Can you work these out from the model? Positions are in its coordinate system, mm. A direction names the side the tool comes from. Give positions to 0.01 mm unless a question says otherwise; leave off trailing zeros. Order: outer loops, then holes, each group sorted by start corner. A loop starts at its lowest first (then second) coordinate and runs counter-clockwise, first axis right, second up. Notation, with made-up numbers: (56.25, 50.25) -> (105.25, 50.25) arc R26 cw to (105.25, 83.25) -> close; hole circle Ø7 at (57.5, 79.5). An arc over 180 degrees is marked (long way). Answer as a JSON object with one key per item and string values.
```python
from build123d import *

# Parameters (mm, degrees)
SKETCH1_W                       = 24.8412
SKETCH1_H                       = 46.101
SKETCH1_R                       = 2.6416
BOSS_EXTRUDE1_DEPTH             = 2.54
BOSS_EXTRUDE2_REACH             = 28.307
SKETCH2_R                       = 3.175
BOSS_EXTRUDE2_DIRECTION_2_REACH = 28.307
CUT_EXTRUDE1_DEPTH              = 46.500059073
CUT_EXTRUDE1_DEPTH_BACK         = 46.500059073
SKETCH3_W                       = 19.7612
SKETCH3_H                       = 34.671
FILLET1_R                       = 2.54


with BuildPart() as part:
    # Sketch1 → Boss-Extrude1 (new body)
    with BuildSketch(Plane(origin=(0, 0, 0), x_dir=(1, 0, 0), z_dir=(0, 1, 0))):
        Rectangle(SKETCH1_W, SKETCH1_H)
        with Locations(Location((-8.255, 17.9959, 0), (0, 0, 270))):
            Circle(SKETCH1_R, mode=Mode.SUBTRACT)
        with Locations(Location((8.255, 17.9959, 0), (0, 0, 270))):
            Circle(SKETCH1_R, mode=Mode.SUBTRACT)
        with Locations(Location((8.255, -17.9959, 0), (0, 0, 270))):
            Circle(SKETCH1_R, mode=Mode.SUBTRACT)
        with Locations(Location((-8.255, -17.9959, 0), (0, 0, 270))):
            Circle(SKETCH1_R, mode=Mode.SUBTRACT)
    extrude(amount=-BOSS_EXTRUDE1_DEPTH)

    # Boss-Extrude2: up to this face of the body (flat: up to its plane)
    boss_extrude2_end = Plane(part.part.faces().sort_by_distance((12.4206, -1.27, 0))[0])
    # Sketch2 → Boss-Extrude2 (add, up to the picked face)
    with BuildSketch(Plane(origin=(0, 0, 0), x_dir=(0, 0, -1), z_dir=(1, 0, 0)), mode=Mode.PRIVATE) as boss_extrude2_sk1:
        with BuildLine():
            Line((-6.203113115, -32.218898258), (-12.7, -2.54))
            Line((-12.7, -2.54), (12.7, -2.54))
            Line((12.7, -2.54), (6.203113115, -32.218898258))
            ThreePointArc((6.203113115, -32.218898258), (0, -37.211), (-6.203113115, -32.218898258))
        make_face()
        with Locations(Location((0, -30.861, 0), (0, 0, 180))):
            Circle(SKETCH2_R, mode=Mode.SUBTRACT)
    boss_extrude2_tool1 = split(extrude(boss_extrude2_sk1.sketch, amount=BOSS_EXTRUDE2_REACH, mode=Mode.PRIVATE), bisect_by=boss_extrude2_end, keep=Keep.BOTH, mode=Mode.PRIVATE)
    add(boss_extrude2_tool1.solids().sort_by(Axis((0, -16.339772, 0), (1, 0, 0)))[0])

    # Boss-Extrude2 direction 2: up to this face of the body (flat: up to its plane)
    boss_extrude2_direction_2_end = Plane(part.part.faces().sort_by_distance((-12.4206, -1.27, 0))[0])
    # Sketch2 → Boss-Extrude2 direction 2 (add, up to the picked face)
    with BuildSketch(Plane(origin=(0, 0, 0), x_dir=(0, 0, -1), z_dir=(1, 0, 0)), mode=Mode.PRIVATE) as boss_extrude2_direction_2_sk1:
        with BuildLine():
            Line((-6.203113115, -32.218898258), (-12.7, -2.54))
            Line((-12.7, -2.54), (12.7, -2.54))
            Line((12.7, -2.54), (6.203113115, -32.218898258))
            ThreePointArc((6.203113115, -32.218898258), (0, -37.211), (-6.203113115, -32.218898258))
        make_face()
        with Locations(Location((0, -30.861, 0), (0, 0, 180))):
            Circle(SKETCH2_R, mode=Mode.SUBTRACT)
    boss_extrude2_direction_2_tool1 = split(extrude(boss_extrude2_direction_2_sk1.sketch, amount=-BOSS_EXTRUDE2_DIRECTION_2_REACH, mode=Mode.PRIVATE), bisect_by=boss_extrude2_direction_2_end, keep=Keep.BOTH, mode=Mode.PRIVATE)
    add(boss_extrude2_direction_2_tool1.solids().sort_by(Axis((0, -16.339772, 0), (-1, 0, 0)))[0])

    # Sketch3 → Cut-Extrude1 (cut, two sides: drawn at the far end of the back side and taken through both)
    with BuildSketch(Plane.XY.offset(-CUT_EXTRUDE1_DEPTH_BACK)):
        with Locations((0, -19.8755)):
            Rectangle(SKETCH3_W, SKETCH3_H)
    extrude(amount=CUT_EXTRUDE1_DEPTH + CUT_EXTRUDE1_DEPTH_BACK, mode=Mode.SUBTRACT)

    # Fillet1
    fillet1_edges = [part.edges().sort_by_distance(p)[0] for p in [
        (-9.8806, -2.54, 0),
        (9.8806, -2.54, 0),
        (-12.4206, -1.27, -23.0505),
        (12.4206, -1.27, -23.0505),
        (12.4206, -1.27, 23.0505),
        (-12.4206, -1.27, 23.0505),
    ]]
    fillet(fillet1_edges, radius=FILLET1_R)


solid = part.part
```
1. Will these pins go through, and if not, where does the flat tip stop? pin 1 Ø1 at (x, z) = (5, 9) entering from +Y; pin 2 Ø2 at (y, z) = (-27, 10) entering from +X; pin 3 Ø6 at (x, z) = (8.26, -18) entering from -Y.
Worked answers:
{"pin 1": "y = 0", "pin 2": "through", "pin 3": "y = -2.54"}
2. If we section it at D-D on z = -5: Please give me the cut outline in (x, y).
Worked answers:
{"outline": "(-12.42, -34.78) -> (-9.88, -34.78) -> (-9.88, -5.08) arc R2.54 cw to (-7.34, -2.54) -> (7.34, -2.54) arc R2.54 cw to (9.88, -5.08) -> (9.88, -34.78) -> (12.42, -34.78) -> (12.42, 0) -> (-12.42, 0) -> close"}
3. If we mould it in two halves opening along Z, with no side actions, what happens to faces 1 (the face through (11.17, -37.21, -0.12)), 2 (the face through (11.045, -17.172, -9.497)), 3 (the face through (8.371, -1.252, -20.635)), 4 (the face through (0, -1, 23.05))? For each: +Z half, -Z half, draft (parallel to the pull), parting line (faces both ways), or undercut.
Worked answers:
{"face 1": "parting line", "face 2": "-Z half", "face 3": "undercut", "face 4": "+Z half"}
4. For faces 5 (the face through (12.421, -14, 0)), 6 (the face through (-9.881, -18, 0)), which set-ups out of +Z, -Z, +X, -X, +Y, -Y let a thin tool reach every point of the face, with its end or its side?
Worked answers:
{"face 5": "+Z, -Z, +X, +Y, -Y", "face 6": "+Z, -Z, -Y"}
5. Please list where these lines run through material, in increasing order: L1, parallel to X at y = -20, z = 8; L2, parallel to Y at x = -11.25, z = 0; L3, parallel to Y at x = 0.5, z = 7.
Worked answers:
{"L1": "-12.42 to -9.88, 9.88 to 12.42", "L2": "-37.21 to -34.04, -27.69 to 0", "L3": "-2.54 to 0"}
6. If we section it at C-C on x = -9: Please give me the cut outline in (y, z).
Worked answers:
{"outline": "(-3.16, -12.56) -> (-2.54, -12.7) -> (-2.54, -15.46) -> (0, -15.46) -> (0, 15.46) -> (-2.54, 15.46) -> (-2.54, 12.7) -> (-3.16, 12.56) -> close; (-2.54, -23.05) -> (0, -23.05) -> (0, -20.53) -> (-2.54, -20.53) -> close; (-2.54, 20.53) -> (0, 20.53) -> (0, 23.05) -> (-2.54, 23.05) -> close"}
7. If we section it at A-A on z = 0: Please give me the cut outline in (x, y).
Worked answers:
{"outline": "(-12.42, -37.21) -> (-9.88, -37.21) -> (-9.88, -34.04) -> (-12.42, -34.04) -> close; (-12.42, -27.69) -> (-9.88, -27.69) -> (-9.88, -5.08) arc R2.54 cw to (-7.34, -2.54) -> (7.34, -2.54) arc R2.54 cw to (9.88, -5.08) -> (9.88, -27.69) -> (12.42, -27.69) -> (12.42, 0) -> (-12.42, 0) -> close; (9.88, -37.21) -> (12.42, -37.21) -> (12.42, -34.04) -> (9.88, -34.04) -> close"}
8. If we section it at B-B on y = -11: Please give me the cut outline in (x, z), then the cut area to 3 significant figures.
Worked answers:
{"outline": "(-12.42, -10.85) -> (-9.88, -10.85) -> (-9.88, 10.85) -> (-12.42, 10.85) -> close; (9.88, -10.85) -> (12.42, -10.85) -> (12.42, 10.85) -> (9.88, 10.85) -> close", "area": "110 mm²"}
